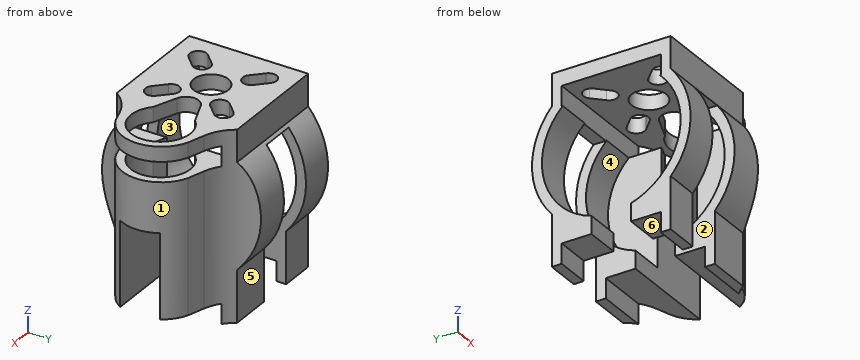
```python
from build123d import *

# Parameters (mm, degrees)
EXTRUDE_DEPTH                             = 50
SKETCH004_AS_DRAWN_R                      = 3.5
EXTRUDE003_DEPTH                          = 16
EXTRUDE003_ONTO_SKETCH004_PLACEMENT_ANGLE = -90
SKETCH002_AS_DRAWN_W                      = 7
SKETCH002_AS_DRAWN_H                      = 55
EXTRUDE002_DEPTH                          = 50
EXTRUDE002_ONTO_SKETCH002_ROLL_ANGLE      = 90
EXTRUDE002_ONTO_SKETCH002_PLACEMENT_ANGLE = 180
SKETCH001_W                               = 20
SKETCH001_H                               = 4
EXTRUDE004_DEPTH                          = 40
CYLINDER_R                                = 14
CYLINDER_DEPTH                            = 21
CYLINDER_PITCH_ANGLE                      = 90
BOX_W                                     = 40
BOX_H                                     = 40
BOX_DEPTH                                 = 38


with BuildPart() as extrude_body:
    # Sketch → Extrude (new body)
    with BuildSketch(Plane.XY.offset(17)):
        with BuildLine():
            ThreePointArc((30.758472, -7.283122), (35.638931, 0), (30.758472, 7.283122))
            Line((30.758472, 7.283122), (27.322862, 8.355563))
            ThreePointArc((21.27771, 16.575411), (22.951713, 11.473701), (27.322862, 8.355563))
            Line((21.27771, 32.499498), (21.27771, 16.575411))
            Line((57.622795, 32.499498), (21.27771, 32.499498))
            Line((57.622795, -32.499498), (57.622795, 32.499498))
            Line((21.27771, -32.499498), (57.622795, -32.499498))
            Line((21.27771, -17.732402), (21.27771, -32.499498))
            ThreePointArc((28.420512, -8.014357), (23.25549, -11.702062), (21.27771, -17.732402))
            Line((30.758472, -7.283122), (28.420512, -8.014357))
        make_face()
    extrude(amount=-EXTRUDE_DEPTH)


with BuildPart() as motor_mount_sketch_extrude:
    # Sketch004 as drawn → Extrude003 (new)
    with BuildSketch(Plane.XY):
        with Locations((0, 15.99875)):
            Circle(SKETCH004_AS_DRAWN_R)
        with BuildLine():
            ThreePointArc((-6.151829, 19.746416), (-3.747666, 19.746416), (-3.747666, 22.150579))
            Line((-3.747666, 22.150579), (-5.868986, 24.271899))
            ThreePointArc((-5.868986, 24.271899), (-8.273149, 24.271899), (-8.273149, 21.867736))
            Line((-6.151829, 19.746416), (-8.273149, 21.867736))
        make_face()
        with BuildLine():
            ThreePointArc((-3.747666, 9.846921), (-3.747666, 12.251084), (-6.151829, 12.251084))
            Line((-6.151829, 12.251084), (-8.273149, 10.129764))
            ThreePointArc((-8.273149, 10.129764), (-8.273149, 7.725601), (-5.868986, 7.725601))
            Line((-3.747666, 9.846921), (-5.868986, 7.725601))
        make_face()
        with BuildLine():
            ThreePointArc((6.151829, 12.251084), (3.747666, 12.251084), (3.747666, 9.846921))
            Line((3.747666, 9.846921), (5.868986, 7.725601))
            ThreePointArc((5.868986, 7.725601), (8.273149, 7.725601), (8.273149, 10.129764))
            Line((6.151829, 12.251084), (8.273149, 10.129764))
        make_face()
        with BuildLine():
            ThreePointArc((3.747666, 22.150579), (3.747666, 19.746416), (6.151829, 19.746416))
            Line((6.151829, 19.746416), (8.273149, 21.867736))
            ThreePointArc((8.273149, 21.867736), (8.273149, 24.271899), (5.868986, 24.271899))
            Line((3.747666, 22.150579), (5.868986, 24.271899))
        make_face()
        with BuildLine():
            Line((-2.424646, 23.060085), (-4.242641, 27.756109))
            ThreePointArc((4.242641, 27.756109), (0, 37.99875), (-4.242641, 27.756109))
            Line((2.424646, 23.060085), (4.242641, 27.756109))
            ThreePointArc((-2.424646, 23.060085), (0, 21.39875), (2.424646, 23.060085))
        make_face()
    extrude(amount=-EXTRUDE003_DEPTH)


with BuildPart() as motor_mount_sketch_extrude_1:
    # Extrude003 onto Sketch004 placement: moved
    add(motor_mount_sketch_extrude.part.moved(Location((-4, 0, 17))).rotate(Axis((-4, 0, 17), (0, 0, 1)), EXTRUDE003_ONTO_SKETCH004_PLACEMENT_ANGLE))


with BuildPart() as side_cute_lite_extrude:
    # Sketch002 as drawn → Extrude002 (new)
    with BuildSketch(Plane.XY):
        with Locations((-10.5, -17.5)):
            Rectangle(SKETCH002_AS_DRAWN_W, SKETCH002_AS_DRAWN_H)
    extrude(amount=-EXTRUDE002_DEPTH)


with BuildPart() as side_cute_lite_extrude_1:
    # Extrude002 onto Sketch002 roll: moved
    add(side_cute_lite_extrude.part.rotate(Axis((0, 0, 0), (1, 0, 0)), EXTRUDE002_ONTO_SKETCH002_ROLL_ANGLE))


with BuildPart() as side_cute_lite_extrude_2:
    # Extrude002 onto Sketch002 placement: moved
    add(side_cute_lite_extrude_1.part.moved(Location((0, 23, 0))).rotate(Axis((0, 23, 0), (0, 0, 1)), EXTRUDE002_ONTO_SKETCH002_PLACEMENT_ANGLE))


with BuildPart() as outer_tube_profile_extrude:
    # Sketch001 → Extrude004 (new body)
    with BuildSketch(Plane(origin=(0, 0, 0), x_dir=(0, -1, 0), z_dir=(-1, 0, 0))):
        with BuildLine():
            Line((-12, 20), (-12, 10.583005))
            ThreePointArc((-12, 10.583005), (-16, 0), (-12, -10.583005))
            Line((-12, -35), (-12, -10.583005))
            Line((-32, -35), (-12, -35))
            Line((-32, 20), (-32, -35))
            Line((-12, 20), (-32, 20))
        make_face()
        with BuildLine():
            ThreePointArc((12, -10.583005), (16, 0), (12, 10.583005))
            Line((12, 20), (12, 10.583005))
            Line((12, 20), (32, 20))
            Line((32, 20), (32, -35))
            Line((32, -35), (12, -35))
            Line((12, -35), (12, -10.583005))
        make_face()
        Polygon((-4, 0), (4, 0), (4, -17), (10, -17), (10, -35), (-10, -35), (-10, -17), (-4, -17), align=None)
        with Locations((0, 12)):
            Rectangle(SKETCH001_W, SKETCH001_H)
    extrude(amount=-EXTRUDE004_DEPTH)


with BuildPart() as cylinder:
    # Cylinder → Cylinder (new body)
    with BuildSketch(Plane.XY):
        Circle(CYLINDER_R)
    extrude(amount=CYLINDER_DEPTH)


with BuildPart() as cylinder_1:
    # Cylinder pitch: moved
    add(cylinder.part.rotate(Axis((0, 0, 0), (0, 1, 0)), CYLINDER_PITCH_ANGLE))


with BuildPart() as cylinder_2:
    # Cylinder placement: moved
    add(cylinder_1.part)


with BuildPart() as cut004:
    # Box → Box (new body)
    with BuildSketch(Plane(origin=(0, -20, -21), x_dir=(1, 0, 0), z_dir=(0, 0, 1))):
        with Locations((20, 20)):
            Rectangle(BOX_W, BOX_H)
    extrude(amount=BOX_DEPTH)

    # Cut: cut Cylinder
    add(cylinder_2.part, mode=Mode.SUBTRACT)

    # Cut001: cut Outer_tube_profile_extrude
    add(outer_tube_profile_extrude.part, mode=Mode.SUBTRACT)

    # Cut002: cut Side_cute_lite_extrude
    add(side_cute_lite_extrude_2.part, mode=Mode.SUBTRACT)

    # Cut003: cut motor_mount_sketch_extrude
    add(motor_mount_sketch_extrude_1.part, mode=Mode.SUBTRACT)

    # Cut004: cut Extrude body
    add(extrude_body.part, mode=Mode.SUBTRACT)


solid = cut004.part
```
Input: part model. Units: mm. Frame: model coordinates. Face numbers are marked on the shaded views. A direction names the side the tool comes from. Give positions to 0.01 mm unless a question says otherwise; leave off trailing zeros. Order: outer loops, then holes, each group sorted by start corner. A loop starts at its lowest first (then second) coordinate and runs counter-clockwise, first axis right, second up. Notation, with made-up numbers: (44, -13.75) - (78, -13.75) arc R34 cw to (78, 16.25) - close; hole circle Ø7 at (46, 2.25). An arc over 180 degrees is marked (long way). One line per item, written item: value.
1. Cut plane D-D, the plane z = 3. Output: boundary loops of the cut face in (x, y), and give its area (3 significant figures).
Determined:
outline: (0, -15.72) - (7, -15.72) - (7, -13.67) - (0, -13.67) - close; (0, 13.67) - (7, 13.67) - (7, 15.72) - (0, 15.72) - close; (14, -15.72) - (21.48, -15.72) arc R10.18 cw to (28.42, -8.01) - (30.76, -7.28) arc R7.87 ccw to (30.76, 7.28) - (27.32, 8.36) arc R8.61 cw to (21.32, 15.72) - (14, 15.72) - (14, 13.67) - (21, 13.67) - (21, 3.18) - (23.76, 4.24) arc R6 cw (long way) to (23.76, -4.24) - (21, -3.18) - (21, -13.67) - (14, -13.67) - close
area: 178 mm2
2. Cut plane B-B, the plane z = -16. Output: boundary loops of the cut face in (x, y).
Determined:
outline: (0, -12) - (7, -12) - (7, -4) - (0, -4) - close; (0, 4) - (7, 4) - (7, 12) - (0, 12) - close; (14, -12) - (23.04, -12) arc R10.18 cw to (28.42, -8.01) - (30.76, -7.28) arc R7.87 ccw to (34.55, -4) - (14, -4) - close; (14, 4) - (34.55, 4) arc R7.87 ccw to (30.76, 7.28) - (27.32, 8.36) arc R8.61 cw to (22.59, 12) - (14, 12) - close
3. Line query: probe 1 along Z at (x, y) = (33, 4.5); probe 2 along Y at (x, z) = (5.5, 13.5); probe 3 along Y at (x, z) = (5, 0). Output: solid intervals per line, ascending.
Determined:
probe 1: -17 to 10, 14 to 17
probe 2: -12 to -10, 10 to 12
probe 3: -16 to -14, 14 to 16
4. Pin query (flat end, axial travel): pin 1 Ø1.2 at (x, z) = (14.5, 12.5) entering from +Y; pin 2 Ø8 at (x, z) = (14, 10.5) entering from +Y; pin 3 Ø12 at (x, z) = (8.5, 12) entering from -Y; pin 4 Ø1 at (y, z) = (3, -12) entering from +X. Return the tip coordinate at first contact, or that it passes through.
Determined:
pin 1: y = 12
pin 2: y = 14.62
pin 3: y = -14.75
pin 4: through
5. Cut plane A-A, the plane y = 0. Output: boundary loops of the cut face in (x, z), and give its area (3 significant figures).
Determined:
outline: (0, 14) - (8.5, 14) - (8.5, 17) - (0, 17) - close; (15.5, 14) - (17.4, 14) - (17.4, 17) - (15.5, 17) - close; (21, 0) - (35.64, 0) - (35.64, 10) - (34, 10) - (34, 1) - (21, 1) - close; (34, 14) - (35.64, 14) - (35.64, 17) - (34, 17) - close
area: 65.5 mm2
6. Reachability of the marked faces 4, 5 and 6 from +Z, -Z, +X, -X, +Y, -Y: full face, straight path, thin tool, end or side. Return the list, or none.
Determined:
face 4: -X
face 5: -Z, +X, -X, +Y
face 6: -Z, +X, -X
7. Cut plane C-C, the plane x = 7.5. Output: boundary loops of the cut face in (y, z).
Determined:
outline: (-12.49, 10) - (-10, 10) - (-10, 14) - (-6.9, 14) - (-6.9, 17) - (-12, 17) - (-12, 10.58) arc R16 ccw to start; (-3.31, 14) - (3.31, 14) - (3.31, 17) - (-3.31, 17) - close; (6.9, 14) - (10, 14) - (10, 10) - (12.49, 10) arc R16 ccw to (12, 10.58) - (12, 17) - (6.9, 17) - close
8. Draft query along X for the marked faces 1, 2 and 3. Return one class per face: released by +X, released by -X, zero draft, split by the parting line, or undercut.
Determined:
face 1: released by +X
face 2: undercut
face 3: zero draft
